Verification items for the finished model (mm, model axes). Face numbers are marked on the shaded views. A direction names the side the tool comes from. Give positions to 0.01 mm unless a question says otherwise; leave off trailing zeros. Order: outer loops, then holes, each group sorted by start corner. A loop starts at its lowest first (then second) coordinate and runs counter-clockwise, first axis right, second up. Notation, with made-up numbers: (30, 70.5) - (89, 70.5) arc R16 ccw to (89, 84.5) - close; hole circle Ø5 at (-17, 22). An arc over 180 degrees is marked (long way). Answer as a JSON object with one key per item and string values. Group by question number.
(1) Mould release check, pull along Y, two halves, no side actions. Record for the marked faces 1, 2 and 3: +Y half, -Y half, draft (parallel to the pull), parting line (faces both ways), or undercut.
(2) Section check C-C (y = 6.5). Record the boundary of the cut face in (x, z) (1 decimal), then the cut area to 3 significant figures.
(3) Section check A-A (x = -17). Record the boundary of the cut face in (y, z) (3 decimals), then the cut area to 3 significant figures.
(4) Depth check by flat-ended pin: pin 1 Ø3.5 at (x, y) = (-41.21, 14.1) entering from +Z; pin 2 Ø2.5 at (x, y) = (30, 4.5) entering from -Z; pin 3 Ø6.5 at (x, y) = (-41.21, -14.1) entering from -Z (3 decimals); pin 4 Ø12 at (x, y) = (20, -13.5) entering from +Z. Enter the tip coordinate at first touch or a pass-through.
(5) Thickness scan on line 1 (X direction, y = -12, z = 17); line 2 (Y direction, x = -40, z = 35.5); line 3 (Z direction, x = -40, y = -3.5) (3 decimals). Record the ranges inside material, lowest first.
(6) Section check B-B (z = 22.5). Record the boundary of the cut face in (x, y).
(7) Access from +Z, -Z, +X, -X, +Y, -Y to the whole of each face (thin tool, end or side, straight path). Record for the marked faces 4 and 5.
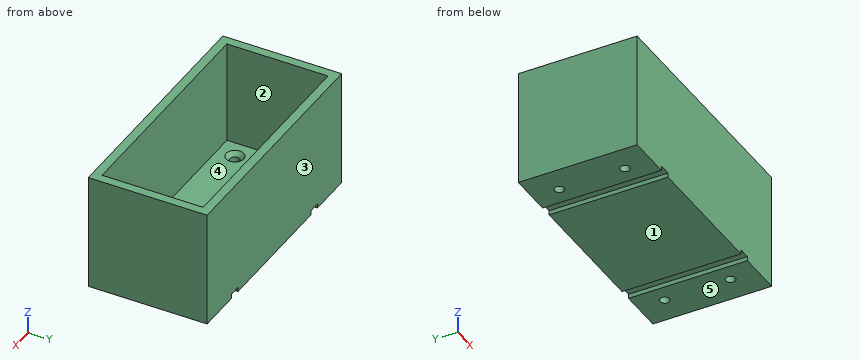
```python
from build123d import *

# Parameters (mm, degrees)
SKETCH001_W      = 97.663
SKETCH001_H      = 43.434
PAD_DEPTH        = 3.81
SKETCH_W         = 105.283
SKETCH_H         = 51.054
SKETCH_W_2       = 97.663
SKETCH_H_2       = 43.434
PAD001_DEPTH     = 48.26
SKETCH003_W      = 19.05
SKETCH003_H      = 51.054
SKETCH003_W_2    = 57.023
PAD002_DEPTH     = 1.905
HOLE_D           = 4.064
HOLE_DEPTH       = 24.9936
HOLE_CSINK_D     = 7.62
HOLE_CSINK_ANGLE = 90


with BuildPart() as part:
    # Sketch001 → Pad (new body)
    with BuildSketch(Plane.XY):
        Rectangle(SKETCH001_W, SKETCH001_H)
    extrude(amount=PAD_DEPTH)

    # Sketch → Pad001 (join)
    with BuildSketch(Plane.XY):
        Rectangle(SKETCH_W, SKETCH_H)
        Rectangle(SKETCH_W_2, SKETCH_H_2, mode=Mode.SUBTRACT)
    extrude(amount=PAD001_DEPTH)

    # Sketch003 → Pad002 (join)
    with BuildSketch(Plane.XY):
        with Locations((-43.1165, 0)):
            Rectangle(SKETCH003_W, SKETCH003_H)
        with Locations((43.1165, 0)):
            Rectangle(SKETCH003_W, SKETCH003_H)
        Rectangle(SKETCH003_W_2, SKETCH003_H)
    extrude(amount=-PAD002_DEPTH)

    # Hole
    with Locations(Plane.XY.offset(3.81)):
        with Locations((41.2115, 14.097), (41.2115, -14.097), (-41.2115, -14.097), (-41.2115, 14.097)):
            CounterSinkHole(HOLE_D / 2, HOLE_CSINK_D / 2, depth=HOLE_DEPTH, counter_sink_angle=HOLE_CSINK_ANGLE)


solid = part.part
```
Solutions:
{
 "1": {"face 1": "draft", "face 2": "undercut", "face 3": "+Y half"},
 "2": {"outline": "(-52.6, -1.9) - (-33.6, -1.9) - (-33.6, 0) - (-28.5, 0) - (-28.5, -1.9) - (28.5, -1.9) - (28.5, 0) - (33.6, 0) - (33.6, -1.9) - (52.6, -1.9) - (52.6, 48.3) - (48.8, 48.3) - (48.8, 3.8) - (-48.8, 3.8) - (-48.8, 48.3) - (-52.6, 48.3) - close", "area": "921 mm2"},
 "3": {"outline": "(-25.527, -1.905) - (25.527, -1.905) - (25.527, 48.26) - (21.717, 48.26) - (21.717, 3.81) - (-21.717, 3.81) - (-21.717, 48.26) - (-25.527, 48.26) - close", "area": "630 mm2"},
 "4": {"pin 1": "passes through", "pin 2": "stops at z = 0", "pin 3": "stops at z = -1.905", "pin 4": "stops at z = 3.81"},
 "5": {"line 1": "x = -52.64 to -48.83, 48.83 to 52.64", "line 2": "y = -25.53 to -21.72, 21.72 to 25.53", "line 3": "z = -1.905 to 3.81"},
 "6": {"outline": "(-52.64, -25.53) - (52.64, -25.53) - (52.64, 25.53) - (-52.64, 25.53) - close; hole (-48.83, -21.72) - (48.83, -21.72) - (48.83, 21.72) - (-48.83, 21.72) - close"},
 "7": {"face 4": "+Z", "face 5": "-Z, +X, -X, +Y, -Y"}
}
